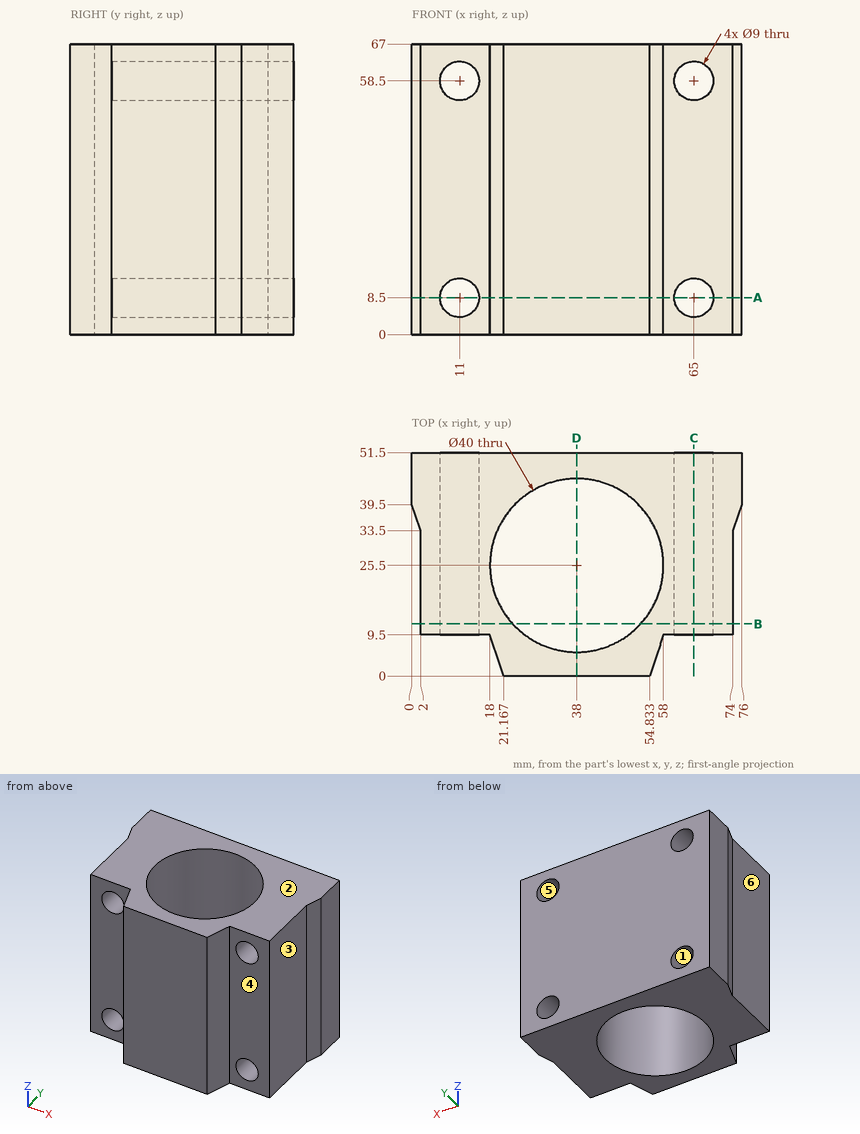
Verification items for this drawing (mm, ordinates from the low corner). A direction names the side the tool comes from. Give positions to 0.01 mm unless a question says otherwise; leave off trailing zeros. Write each loop counter-clockwise with the first axis right and the second up, starting at its lowest first coordinate (ties: lowest second). Pieces come first, ordered by that corner, then holes. Notation, with made-up numbers: M -15.75,66 L 21.25,66 A6 ccw 21.25,77 Z; hole C 59,-15.75 d1. An arc over 180 degrees is marked long. Use one line per item in the form item = value.
(1) Section check B-B on y = 12. Record the boundary of the cut face in (x, z), plus the area to 3 significant figures.
Answer block:
outline = M 2,0 L 23.24,0 L 23.24,67 L 2,67 Z; M 52.76,0 L 74,0 L 74,67 L 52.76,67 Z; hole C 11,8.5 d9; hole C 11,58.5 d9; hole C 65,8.5 d9; hole C 65,58.5 d9
area = 2,590 mm2
(2) Section check A-A on z = 8.5. Record the boundary of the cut face in (x, y), plus the area to 3 significant figures.
Answer block:
outline = M 0,39.5 L 2,33.5 L 2,9.5 L 6.5,9.5 L 6.5,51.5 L 0,51.5 Z; M 15.5,9.5 L 18,9.5 L 21.17,0 L 54.83,0 L 58,9.5 L 60.5,9.5 L 60.5,51.5 L 15.5,51.5 Z; M 69.5,9.5 L 74,9.5 L 74,33.5 L 76,39.5 L 76,51.5 L 69.5,51.5 Z; hole C 38,25.5 d40
area = 1,420 mm2
(3) Section check D-D on x = 38. Record the boundary of the cut face in (y, z).
Answer block:
outline = M 0,0 L 5.5,0 L 5.5,67 L 0,67 Z; M 45.5,0 L 51.5,0 L 51.5,67 L 45.5,67 Z
(4) Tool access check on the marked faces 4, 5 and 6. Record the directions out of +Z, -Z, +X, -X, +Y, -Y that give a thin tool (end or side, any length) a straight path to the whole face; none if there is none.
Answer block:
face_4 = +Z, -Z, +X, -Y
face_5 = +Y, -Y
face_6 = +Z, -Z, -X, -Y
(5) Draft check along X on the marked faces 1, 2 and 3. Enter one of: pulls with the +X half, pulls with the -X half, needs draft (parallel to the pull), parting line crosses it, or undercut.
Answer block:
face_1 = undercut
face_2 = needs draft
face_3 = pulls with the +X half
(6) Section check C-C on x = 65. Record the boundary of the cut face in (y, z), plus the area to 3 significant figures.
Answer block:
outline = M 9.5,0 L 51.5,0 L 51.5,4 L 9.5,4 Z; M 9.5,13 L 51.5,13 L 51.5,54 L 9.5,54 Z; M 9.5,63 L 51.5,63 L 51.5,67 L 9.5,67 Z
area = 2,060 mm2
(7) Material ranges on line 1 along Z through (x, y) = (11, 35); line 2 along Y through (x, z) = (38, 15); line 3 along Z through (x, y) = (13.5, 33), recorded low to high.
Answer block:
line_1 = 0 to 4, 13 to 54, 63 to 67
line_2 = 0 to 5.5, 45.5 to 51.5
line_3 = 0 to 4.76, 12.24 to 54.76, 62.24 to 67
(8) Depth check by flat-ended pin: P1, Ø8, axis at x = 9.5, z = 19.5, coming from the -Y side; P2, Ø7, axis at y = 19.5, z = 49.5, coming from the +X side. Enter the tip coordinate at first touch or a pass-through.
Answer block:
P1 = 9.5
P2 = 74
